from build123d import *

# Parameters (mm, degrees)
SKETCH3_W           = 144.018
SKETCH3_H           = 111.76
BOSS_EXTRUDE2_DEPTH = 5.08
SKETCH5_W           = 6.096
SKETCH5_H           = 4.064
CUT_EXTRUDE1_DEPTH  = 5.08
SKETCH6_W           = 32.512
SKETCH6_H           = 12.7
CUT_EXTRUDE2_DEPTH  = 2.54
SKETCH7_W           = 23.876
SKETCH7_H           = 12.7
CUT_EXTRUDE3_DEPTH  = 2.54


with BuildPart() as part:
    # Sketch3 → Boss-Extrude2 (new body)
    with BuildSketch(Plane(origin=(0, 0, 0), x_dir=(1, 0, 0), z_dir=(0, 1, 0))):
        with Locations((-10.674968857, -20.111055569)):
            Rectangle(SKETCH3_W, SKETCH3_H)
    extrude(amount=BOSS_EXTRUDE2_DEPTH)

    # Sketch5 → Cut-Extrude1 (cut)
    with BuildSketch(Plane(origin=(0, 5.08, 0), x_dir=(1, 0, 0), z_dir=(0, 1, 0))):
        with Locations((-74.544129387, 31.450944431)):
            Rectangle(SKETCH5_W, SKETCH5_H)
        with Locations((54.476031143, 31.450944431)):
            Rectangle(SKETCH5_W, SKETCH5_H)
        with Locations((-15.53142752, -71.419055569)):
            Rectangle(SKETCH5_W, SKETCH5_H)
    extrude(amount=-CUT_EXTRUDE1_DEPTH, mode=Mode.SUBTRACT)

    # Sketch6 → Cut-Extrude2 (cut)
    with BuildSketch(Plane(origin=(0, 5.08, 0), x_dir=(1, 0, 0), z_dir=(0, 1, 0))):
        with Locations((-10.674968857, -14.750552476)):
            Rectangle(SKETCH6_W, SKETCH6_H)
    extrude(amount=-CUT_EXTRUDE2_DEPTH, mode=Mode.SUBTRACT)

    # Sketch7 → Cut-Extrude3 (cut)
    with BuildSketch(Plane(origin=(0, 2.54, 0), x_dir=(1, 0, 0), z_dir=(0, 1, 0))):
        with Locations((-10.928968857, -14.750552476)):
            Rectangle(SKETCH7_W, SKETCH7_H)
    extrude(amount=-CUT_EXTRUDE3_DEPTH, mode=Mode.SUBTRACT)


solid = part.part
For this review, take the finished solid that the model builds, in its own axes (mm). A direction names the side the tool comes from. Round coordinates to 2 decimals unless told otherwise and drop trailing zeros. Loops run counter-clockwise (first coordinate to the right, second up) from the corner with the lowest first, then second, coordinate; pieces in that order, holes last. Notation, with made-up numbers: (39, 16.5) - (85, 16.5) arc R22 cw to (85, 55.5) - close; hole circle Ø6 at (-12.5, 55). An arc over 180 degrees is marked (long way). Use one line per item in the form item = value.
1) We need section A-A on x = -9.5. Write out the cut boundary in (y, z).
Solutions:
outline = (0, -35.77) - (5.08, -35.77) - (5.08, 8.4) - (0, 8.4) - close; (0, 21.1) - (5.08, 21.1) - (5.08, 75.99) - (0, 75.99) - close
2) Wall thickness on probe 1 along X at (y, z) = (2.4, 70.5); probe 2 along X at (y, z) = (0.4, 13); probe 3 along Z at (x, y) = (2.5, 4.55): over which ranges is each line inside the solid? List them lowest first.
Solutions:
probe_1 = -82.68 to -18.58, -12.48 to 61.33
probe_2 = -82.68 to -22.87, 1.01 to 61.33
probe_3 = -35.77 to 8.4, 21.1 to 75.99
3) Mouldability with a two-part tool opening along Z and no side actions: class faces 1 (the face through (-12, 3, 75.991)), 2 (the face through (-77.592, 3, -31)), 3 (the face through (-82.684, 3, 21)), 4 (the face through (-16, 3, 69.387)) as pulls with the +Z half, pulls with the -Z half, needs draft (parallel to the pull), parting line crosses it, or undercut.
Solutions:
face_1 = pulls with the +Z half
face_2 = undercut
face_3 = needs draft
face_4 = undercut
4) Tool access review of faces 5 (the face through (-12, 0, 32)), 6 (the face through (-11, 3, 8.401)), 7 (the face through (54, 3, -29.419)): name each direction out of +Z, -Z, +X, -X, +Y, -Y from which nothing blocks a thin tool from reaching the whole face with its end or side.
Solutions:
face_5 = +Z, -Z, +X, -X, -Y
face_6 = +Y
face_7 = +Y, -Y
5) We need section B-B on y = 3.6. Write out the cut boundary in (x, z), then the cut area to 3 significant figures.
Solutions:
outline = (-82.68, -35.77) - (61.33, -35.77) - (61.33, 75.99) - (-82.68, 75.99) - close; hole (-77.59, -33.48) - (-71.5, -33.48) - (-71.5, -29.42) - (-77.59, -29.42) - close; hole (-26.93, 8.4) - (5.58, 8.4) - (5.58, 21.1) - (-26.93, 21.1) - close; hole (-18.58, 69.39) - (-12.48, 69.39) - (-12.48, 73.45) - (-18.58, 73.45) - close; hole (51.43, -33.48) - (57.52, -33.48) - (57.52, -29.42) - (51.43, -29.42) - close
area = 15,600 mm2
